Could you check a few things on this model? Use its own coordinates, in mm. A direction names the side the tool comes from. Round coordinates to 2 decimals unless told otherwise and drop trailing zeros. Order: outer loops, then holes, each group sorted by start corner. A loop starts at its lowest first (then second) coordinate and runs counter-clockwise, first axis right, second up.
```python
from build123d import *

# Parameters (mm, degrees)
SZKIC1_W                         = 222
SZKIC1_H                         = 125
SZKIC1_R                         = 13
SZKIC1_R_2                       = 4
DODANIE_WYCI_GNI_CIE1_DEPTH      = 13.5
DODANIE_WYCI_GNI_CIE1_DEPTH_BACK = 13.5
SZKIC4_W                         = 15
SZKIC4_H                         = 27
DODANIE_WYCI_GNI_CIE4_DEPTH      = 36
SZKIC13_R                        = 38.75
WYTNIJ_WYCI_GNI_CIE4_DEPTH       = 17
SZKIC15_R                        = 44.5
WYTNIJ_WYCI_GNI_CIE5_DEPTH       = 5
POCHYLENIE1_ANGLE                = 45
SZKIC16_R                        = 13
SZKIC16_R_2                      = 4
DODANIE_WYCI_GNI_CIE6_DEPTH      = 21
SZKIC5_R                         = 6
WYTNIJ_WYCI_GNI_CIE3_DEPTH       = 223
WYTNIJ_WYCI_GNI_CIE6_DEPTH       = 49
ZAOKR_GLENIE1_R                  = 30
ZAOKR_GLENIE2_R                  = 30
SZKIC19_W                        = 40
SZKIC19_H                        = 60
DODANIE_WYCI_GNI_CIE7_DEPTH      = 48
WYTNIJ_WYCI_GNI_CIE7_REACH       = 133
SZKIC23_R                        = 20
WYTNIJ_WYCI_GNI_CIE8_REACH       = 50
ZAOKR_GLENIE4_R                  = 5
ZAOKR_GLENIE5_R                  = 5
WYTNIJ_WYCI_GNI_CIE9_DEPTH       = 48
OTW_R_GWINTOWANY_M81_AT_2_COUNT  = 2
OTW_R_GWINTOWANY_M81_AT_2_PITCH  = 26
OTW_R_GWINTOWANY_M82_AT_2_COUNT  = 2
OTW_R_GWINTOWANY_M82_AT_2_PITCH  = 26


with BuildPart() as part:
    # Szkic1 → Dodanie-wyci_gni_cie1 (new body, two sides)
    with BuildSketch(Plane.XY) as dodanie_wyci_gni_cie1_sk:
        Rectangle(SZKIC1_W, SZKIC1_H)
        Circle(SZKIC1_R, mode=Mode.SUBTRACT)
        with Locations((-32, 0)):
            Circle(SZKIC1_R_2, mode=Mode.SUBTRACT)
        with Locations((-16, 27.712812921)):
            Circle(SZKIC1_R_2, mode=Mode.SUBTRACT)
        with Locations((16, 27.712812921)):
            Circle(SZKIC1_R_2, mode=Mode.SUBTRACT)
        with Locations((32, 0)):
            Circle(SZKIC1_R_2, mode=Mode.SUBTRACT)
        with Locations((16, -27.712812921)):
            Circle(SZKIC1_R_2, mode=Mode.SUBTRACT)
        with Locations((-16, -27.712812921)):
            Circle(SZKIC1_R_2, mode=Mode.SUBTRACT)
    extrude(amount=DODANIE_WYCI_GNI_CIE1_DEPTH)
    extrude(dodanie_wyci_gni_cie1_sk.sketch, amount=-DODANIE_WYCI_GNI_CIE1_DEPTH_BACK)

    # Szkic4 → Dodanie-wyci_gni_cie4 (add)
    with BuildSketch(Plane(origin=(0, 62.5, 0), x_dir=(1, 0, 0), z_dir=(0, 1, 0))):
        with Locations((-103.5, 0)):
            Rectangle(SZKIC4_W, SZKIC4_H)
        with Locations((-53.5, 0)):
            Rectangle(SZKIC4_W, SZKIC4_H)
        with Locations((53.5, 0)):
            Rectangle(SZKIC4_W, SZKIC4_H)
        with Locations((103.5, 0)):
            Rectangle(SZKIC4_W, SZKIC4_H)
    extrude(amount=DODANIE_WYCI_GNI_CIE4_DEPTH)

    # Szkic13 → Wytnij-wyci_gni_cie4 (cut)
    with BuildSketch(Plane.XY.offset(13.5)):
        Circle(SZKIC13_R)
    extrude(amount=-WYTNIJ_WYCI_GNI_CIE4_DEPTH, mode=Mode.SUBTRACT)

    # Szkic15 → Wytnij-wyci_gni_cie5 (cut)
    with BuildSketch(Plane.XY.offset(13.5)):
        Circle(SZKIC15_R)
    extrude(amount=-WYTNIJ_WYCI_GNI_CIE5_DEPTH, mode=Mode.SUBTRACT)

    # Pochylenie1
    pochylenie1_faces = [part.faces().sort_by_distance(p)[0] for p in [
        (-44.5, 0, 11),
    ]]
    draft(pochylenie1_faces, Plane.XY.offset(8.5), POCHYLENIE1_ANGLE)

    # Szkic16 → Dodanie-wyci_gni_cie6 (add)
    with BuildSketch(Plane(origin=(0, 0, -13.5), x_dir=(-1, 0, 0), z_dir=(0, 0, -1))):
        Polygon((-111, 98.5), (-111, -62.5), (111, -62.5), (111, 98.5), (96, 98.5), (96, 62.5), (61, 62.5), (61, 98.5), (46, 98.5), (46, 62.5), (-46, 62.5), (-46, 98.5), (-61, 98.5), (-61, 62.5), (-96, 62.5), (-96, 98.5), align=None)
        Circle(SZKIC16_R, mode=Mode.SUBTRACT)
        with Locations((32, 0)):
            Circle(SZKIC16_R_2, mode=Mode.SUBTRACT)
        with Locations((16, 27.712812921)):
            Circle(SZKIC16_R_2, mode=Mode.SUBTRACT)
        with Locations((-16, 27.712812921)):
            Circle(SZKIC16_R_2, mode=Mode.SUBTRACT)
        with Locations((-32, 0)):
            Circle(SZKIC16_R_2, mode=Mode.SUBTRACT)
        with Locations((-16, -27.712812921)):
            Circle(SZKIC16_R_2, mode=Mode.SUBTRACT)
        with Locations((16, -27.712812921)):
            Circle(SZKIC16_R_2, mode=Mode.SUBTRACT)
    extrude(amount=DODANIE_WYCI_GNI_CIE6_DEPTH)

    # Szkic5 → Wytnij-wyci_gni_cie3 (cut, through all)
    with BuildSketch(Plane.ZY.offset(111)):
        with Locations((-10.5, 78.5)):
            Circle(SZKIC5_R)
    extrude(amount=-WYTNIJ_WYCI_GNI_CIE3_DEPTH, mode=Mode.SUBTRACT)

    # Szkic18 → Wytnij-wyci_gni_cie6 (cut, through all)
    with BuildSketch(Plane(origin=(0, 0, -34.5), x_dir=(-1, 0, 0), z_dir=(0, 0, -1))):
        Polygon((111, 22.5), (46, -62.5), (111, -62.5), align=None)
        Polygon((-111, -62.5), (-46, -62.5), (-111, 22.5), align=None)
    extrude(amount=-WYTNIJ_WYCI_GNI_CIE6_DEPTH, mode=Mode.SUBTRACT)

    # Zaokr_glenie1
    zaokr_glenie1_edges = [part.edges().sort_by_distance(p)[0] for p in [
        (-111, 22.5, -10.5),
    ]]
    fillet(zaokr_glenie1_edges, radius=ZAOKR_GLENIE1_R)

    # Zaokr_glenie2
    zaokr_glenie2_edges = [part.edges().sort_by_distance(p)[0] for p in [
        (-46, -62.5, -10.5),
        (111, 22.5, -10.5),
        (46, -62.5, -10.5),
    ]]
    fillet(zaokr_glenie2_edges, radius=ZAOKR_GLENIE2_R)

    # Szkic19 → Dodanie-wyci_gni_cie7 (add)
    with BuildSketch(Plane(origin=(0, 0, -34.5), x_dir=(-1, 0, 0), z_dir=(0, 0, -1))):
        with Locations((0, -92.5)):
            Rectangle(SZKIC19_W, SZKIC19_H)
    extrude(amount=-DODANIE_WYCI_GNI_CIE7_DEPTH)

    # Szkic23 → Wytnij-wyci_gni_cie7 (cut, up to next)
    with BuildSketch(Plane(origin=(20, 0, 0), x_dir=(0, 0, -1), z_dir=(1, 0, 0)), mode=Mode.PRIVATE) as wytnij_wyci_gni_cie7_sk1:
        with Locations((10.5, -92.5)):
            Circle(SZKIC23_R)
    wytnij_wyci_gni_cie7_tool1 = extrude(wytnij_wyci_gni_cie7_sk1.sketch, amount=-WYTNIJ_WYCI_GNI_CIE7_REACH, mode=Mode.PRIVATE) & part.part
    add(wytnij_wyci_gni_cie7_tool1.solids().sort_by_distance((20, -92.5, -10.5))[0], mode=Mode.SUBTRACT)

    # Szkic24 → Wytnij-wyci_gni_cie8 (cut, up to next)
    with BuildSketch(Plane(origin=(0, 0, -34.5), x_dir=(-1, 0, 0), z_dir=(0, 0, -1)), mode=Mode.PRIVATE) as wytnij_wyci_gni_cie8_sk1:
        with BuildLine():
            Line((-96, 62.5), (-61, 62.5))
            ThreePointArc((-61, 62.5), (-78.5, 45), (-96, 62.5))
        make_face()
    wytnij_wyci_gni_cie8_tool1 = extrude(wytnij_wyci_gni_cie8_sk1.sketch, amount=-WYTNIJ_WYCI_GNI_CIE8_REACH, mode=Mode.PRIVATE) & part.part
    add(wytnij_wyci_gni_cie8_tool1.solids().sort_by_distance((78.5, 55.072769, -34.5))[0], mode=Mode.SUBTRACT)
    # Szkic24 → Wytnij-wyci_gni_cie8 (cut, up to next)
    with BuildSketch(Plane(origin=(0, 0, -34.5), x_dir=(-1, 0, 0), z_dir=(0, 0, -1)), mode=Mode.PRIVATE) as wytnij_wyci_gni_cie8_sk2:
        with BuildLine():
            Line((61, 62.5), (96, 62.5))
            ThreePointArc((96, 62.5), (78.5, 45), (61, 62.5))
        make_face()
    wytnij_wyci_gni_cie8_tool2 = extrude(wytnij_wyci_gni_cie8_sk2.sketch, amount=-WYTNIJ_WYCI_GNI_CIE8_REACH, mode=Mode.PRIVATE) & part.part
    add(wytnij_wyci_gni_cie8_tool2.solids().sort_by_distance((-78.5, 55.072769, -34.5))[0], mode=Mode.SUBTRACT)

    # Zaokr_glenie4
    zaokr_glenie4_edges = [part.edges().sort_by_distance(p)[0] for p in [
        (20, -62.5, -10.5),
        (-20, -62.5, -10.5),
    ]]
    fillet(zaokr_glenie4_edges, radius=ZAOKR_GLENIE4_R)

    # Zaokr_glenie5
    zaokr_glenie5_edges = [part.edges().sort_by_distance(p)[0] for p in [
        (0, -122.5, -34.5),
        (0, -122.5, 13.5),
    ]]
    fillet(zaokr_glenie5_edges, radius=ZAOKR_GLENIE5_R)

    # Szkic25 → Wytnij-wyci_gni_cie9 (cut)
    with BuildSketch(Plane.XY.offset(13.5)):
        with BuildLine():
            Line((-60.951491344, -10.353512592), (-74.069286372, 21.36621852))
            ThreePointArc((-74.069286372, 21.36621852), (-84.742802137, 24.999340902), (-86.957683747, 13.944124193))
            Line((-86.957683747, 13.944124193), (-66.106850294, -13.322350323))
            ThreePointArc((-66.106850294, -13.322350323), (-62.22665594, -14.099736361), (-60.951491344, -10.353512592))
        make_face()
        with BuildLine():
            Line((66.106850294, -13.322350323), (86.957683747, 13.944124193))
            ThreePointArc((86.957683747, 13.944124193), (84.742802137, 24.999340902), (74.069286372, 21.36621852))
            Line((74.069286372, 21.36621852), (60.951491344, -10.353512592))
            ThreePointArc((60.951491344, -10.353512592), (62.22665594, -14.099736361), (66.106850294, -13.322350323))
        make_face()
    extrude(amount=-WYTNIJ_WYCI_GNI_CIE9_DEPTH, mode=Mode.SUBTRACT)

    # Szkic28 → Otw_r gwintowany M81 (revolve, cut)
    with BuildSketch(Plane(origin=(-92.067147824, -2.258345153, -20.15), x_dir=(0.607450108, -0.794357833, 0), z_dir=(0, 0, 1))):
        Polygon((0, 0), (0, 47.042926105), (3.4, 45), (3.4, 0), align=None)
    otw_r_gwintowany_m81 = revolve(axis=Axis((-97.111320063, -6.115653336, -20.15), (0.794357833, 0.607450108, 0)), mode=Mode.SUBTRACT)

    # Otw_r gwintowany M81 at 2: Otw_r gwintowany M81 ×2
    with Locations(*[Vector(-0.233634657, 0.305522243, 0.923076923) * (i * OTW_R_GWINTOWANY_M81_AT_2_PITCH) for i in range(1, OTW_R_GWINTOWANY_M81_AT_2_COUNT)]):
        add(otw_r_gwintowany_m81, mode=Mode.SUBTRACT)

    # Szkic30 → Otw_r gwintowany M82 (revolve, cut)
    with BuildSketch(Plane(origin=(-61.694642445, -41.976236802, 3.85), x_dir=(0.607450108, -0.794357833, 0), z_dir=(0, 0, 1))):
        Polygon((0, 0), (0, 27.042926105), (3.4, 25), (3.4, 0), align=None)
    otw_r_gwintowany_m82 = revolve(axis=Axis((-66.738814685, -45.833544985, 3.85), (0.794357833, 0.607450108, 0)), mode=Mode.SUBTRACT)

    # Otw_r gwintowany M82 at 2: Otw_r gwintowany M82 ×2
    with Locations(*[Vector(-0.233634657, 0.305522243, -0.923076923) * (i * OTW_R_GWINTOWANY_M82_AT_2_PITCH) for i in range(1, OTW_R_GWINTOWANY_M82_AT_2_COUNT)]):
        add(otw_r_gwintowany_m82, mode=Mode.SUBTRACT)

    # Lustro1: Otw_r gwintowany M82, Otw_r gwintowany M81 across plane
    add(otw_r_gwintowany_m82.mirror(Plane(origin=(0, 0, 0), x_dir=(0, 0, 1), z_dir=(1, 0, 0))), mode=Mode.SUBTRACT)
    add(otw_r_gwintowany_m81.mirror(Plane(origin=(0, 0, 0), x_dir=(0, 0, 1), z_dir=(1, 0, 0))), mode=Mode.SUBTRACT)

    # Lustro1 copy 1 sketch → Lustro1 copy 1 (revolve, cut)
    with BuildSketch(Plane(origin=(67.769143521, -34.032658472, -20.15), x_dir=(-0.607450108, -0.794357833, 0), z_dir=(0, 0, 1))):
        Polygon((0, 0), (0, -27.042926105), (3.4, -25), (3.4, 0), align=None)
    revolve(axis=Axis((72.813315761, -37.889966655, -20.15), (0.794357833, -0.607450108, 0)), mode=Mode.SUBTRACT)

    # Lustro1 copy 2 sketch → Lustro1 copy 2 (revolve, cut)
    with BuildSketch(Plane(origin=(98.1416489, 5.685233176, 3.85), x_dir=(-0.607450108, -0.794357833, 0), z_dir=(0, 0, 1))):
        Polygon((0, 0), (0, -47.042926105), (3.4, -45), (3.4, 0), align=None)
    revolve(axis=Axis((103.185821139, 1.827924993, 3.85), (0.794357833, -0.607450108, 0)), mode=Mode.SUBTRACT)


solid = part.part
```
Q1. For faces 4 (the cylindrical face through (-8.4, -37.83, 2.58)), 5 (the flat face through (67.602, 5.728, -10.164)), 6 (the flat face through (20, -114, -11)), 7 (the cylindrical face through (-67.3, 25.2, 2.8)), which set-ups out of +Z, -Z, +X, -X, +Y, -Y let a thin tool reach every point of the face, with its end or its side?
Q2. We'd pull the mould along Y, two halves only. Please class faces 1 (the cylindrical face through (44.29, -59.48, -10.16)), 2 (the cylindrical face through (-94.39, 12.83, 3.7)), 3 (the cylindrical face through (78.115, 45.004, -10.836)): released by +Y, released by -Y, zero draft, split by the parting line, or undercut.
Q3. For P1, Ø9, axis at x = -32, y = 0, coming from the +Z side; P2, Ø6, axis at x = 78, z = -25, coming from the -Y side; P3, Ø8, axis at y = 6, z = -3, coming from the +X side, each with a flat end and sliding along its axis, tell me the tip position at first contact or that it passes through.
Q4. I need wall thicknesses on L1, parallel to Y at x = -16, z = -9; L2, parallel to Y at x = 32.5, z = -21.5; L3, parallel to X at y = 84.5, z = -2. Which ranges of each line are inside material? Lowest first, please.
Q5. Imagine slicing it at B-B, the plane y = -76. Please give me the cut outline in (x, z).
Q6. Imagine slicing it at A-A, the plane x = 0. Please give me the cut outline in (y, z), then the cut area to 3 significant figures.
Filled in:
1. face 4: +Z
1. face 5: +Z, -Z
1. face 6: +Z, -Z, +X, -Y
1. face 7: none
2. face 1: released by -Y
2. face 2: undercut
2. face 3: released by +Y
3. P1: stops at z = -3.5
3. P2: stops at y = -24.58
3. P3: stops at x = 101.44
4. L1: y = -122.5 to -112.44, -72.56 to -31.71, -23.71 to 23.71, 31.71 to 62.5
4. L2: y = -62.47 to -3.97, 3.97 to 62.5
4. L3: x = -111 to -96, -61 to -46, 46 to 61, 96 to 111
5. outline: (-20, -34.5) - (20, -34.5) - (20, -21.8) - (-20, -21.8) - close; (-20, 0.8) - (20, 0.8) - (20, 13.5) - (-20, 13.5) - close
6. outline: (-122.5, -29.5) arc R5 ccw to (-117.5, -34.5) - (-13, -34.5) - (-13, -3.5) - (-38.75, -3.5) - (-38.75, 8.5) - (-44.5, 8.5) - (-49.5, 13.5) - (-117.5, 13.5) arc R5 ccw to (-122.5, 8.5) - close; (13, -34.5) - (62.5, -34.5) - (62.5, 13.5) - (49.5, 13.5) - (44.5, 8.5) - (38.75, 8.5) - (38.75, -3.5) - (13, -3.5) - close; hole circle Ø40 at (-92.5, -10.5)
6. area: 5,410 mm2
